```python
from build123d import *

# Parameters (mm, degrees)
SKETCH1_R          = 22
SKETCH1_R_2        = 19
OUTER_RING_DEPTH   = 8
SKETCH2_R          = 15
SKETCH2_R_2        = 9.25
HUB_DEPTH          = 8
SKETCH3_W          = 6
SKETCH3_H          = 5
SPOKES_DEPTH       = 8
SKETCH4_R          = 11
BEARING_SEAT_DEPTH = 7
SCREW_GROOVE_DEPTH = 2


with BuildPart() as part:
    # Sketch1 → Outer_ring (new body)
    with BuildSketch(Plane.XY):
        Circle(SKETCH1_R)
        Circle(SKETCH1_R_2, mode=Mode.SUBTRACT)
    extrude(amount=OUTER_RING_DEPTH)



with BuildPart() as body_2:
    # Sketch2 → Hub (new body)
    with BuildSketch(Plane.XY):
        Circle(SKETCH2_R)
        Circle(SKETCH2_R_2, mode=Mode.SUBTRACT)
    extrude(amount=HUB_DEPTH)


with BuildPart() as part_1:
    add(part.part)

    add(body_2.part)  # Spokes merges body 2
    # Sketch3 → Spokes (add)
    with BuildSketch(Plane.XY):
        Polygon((9.165063509, 10.874355653), (12.165063509, 16.070508076), (7.834936491, 18.570508076), (4.834936491, 13.374355653), align=None)
        with Locations((-17, 0)):
            Rectangle(SKETCH3_W, SKETCH3_H)
        Polygon((4.834936491, -13.374355653), (7.834936491, -18.570508076), (12.165063509, -16.070508076), (9.165063509, -10.874355653), align=None)
    extrude(amount=SPOKES_DEPTH)

    # Sketch4 → Bearing_seat (cut)
    with BuildSketch(Plane.XY):
        Circle(SKETCH4_R)
    extrude(amount=BEARING_SEAT_DEPTH, mode=Mode.SUBTRACT)

    # Sketch5 → Screw_groove (cut)
    with BuildSketch(Plane.XY.offset(3)):
        Polygon((20.820342089, -2.741050037), (20.849003007, -2.513776761), (20.875183103, -2.286204372), (20.89887926, -2.058359947), (20.92008866, -1.830270598), (20.938808778, -1.601963465), (20.955037388, -1.373465714), (20.968772558, -1.144804534), (20.980012653, -0.916007135), (20.988756337, -0.687100739), (20.995002569, -0.458112586), (20.998750605, -0.229069921), (21, 0), (20.998750605, 0.229069921), (20.995002569, 0.458112586), (20.988756337, 0.687100739), (20.980012653, 0.916007135), (20.968772558, 1.144804534), (20.955037388, 1.373465714), (20.938808778, 1.601963465), (20.92008866, 1.830270598), (20.89887926, 2.058359947), (20.875183103, 2.286204372), (20.849003007, 2.513776761), (20.820342089, 2.741050037), (23.298954242, 3.067365517), (23.298954242, -3.067365517), align=None)
    extrude(amount=SCREW_GROOVE_DEPTH, mode=Mode.SUBTRACT)


solid = part_1.part
```
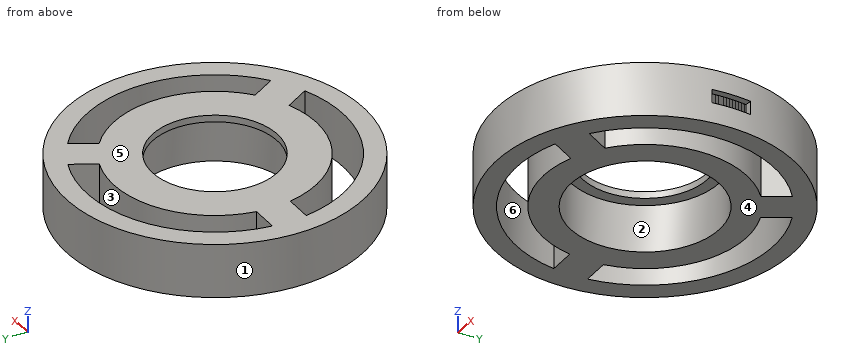
Here's how the part is built. I have some questions about the finished solid (model axes, mm). Face numbers are marked on the shaded views. A direction names the side the tool comes from. Give positions to 0.01 mm unless a question says otherwise; leave off trailing zeros. Order: outer loops, then holes, each group sorted by start corner. A loop starts at its lowest first (then second) coordinate and runs counter-clockwise, first axis right, second up. Notation, with made-up numbers: M 53.25,75 L 70.25,75 A21 ccw 70.25,112 Z; hole C 25.5,-24.75 d10. An arc over 180 degrees is marked long. Use a Markdown table: item, result. Add a question column.
1. If we mould it in two halves opening along Y, with no side actions, what happens to the marked faces 1, 2, 3 and 4? For each: +Y half, -Y half, draft (parallel to the pull), parting line (faces both ways), or undercut.
2. For pin 1 Ø2 at (x, z) = (-16.5, 2) entering from -Y; pin 2 Ø1.5 at (x, y) = (1.5, -9.5) entering from -Z; pin 3 Ø1 at (y, z) = (-15, 3) entering from +X; pin 4 Ø12 at (x, y) = (9, 2) entering from +Z, each with a flat end and sliding along its axis, tell me the tip position at first contact or that it passes through.
3. Suppose I cut it at C-C (y = -5.5). List the corners of the cut face in (x, z) for me.
4. Suppose I cut it at B-B (z = 6). List the corners of the cut face in (x, y) for me, and give its area (3 significant figures).
5. Suppose I cut it at A-A (x = 0). List the corners of the cut face in (y, z) for me.
6. On a 3-axis mill with a long thin cutter (end or side, diameter ignored), from which of +Z, -Z, +X, -X, +Y, -Y can I reach the whole of each face in a straight line? I mean the marked faces 5 and 6. Say none if no direction works.
7. I need wall thicknesses on probe 1 along Y at (x, z) = (0, 7.5); probe 2 along Y at (x, z) = (0, 3.75); probe 3 along Y at (x, z) = (-12.5, 5.75). Which ranges of each line are inside material? Lowest first, please. Write a range as from..to.
Results list:
| question | item | result |
|---|---|---|
| 1 | face 1 | parting line |
| 1 | face 2 | undercut |
| 1 | face 3 | undercut |
| 1 | face 4 | draft |
| 2 | pin 1 | stops at y = -15.61 |
| 2 | pin 2 | stops at z = 7 |
| 2 | pin 3 | stops at x = 16.55 |
| 2 | pin 4 | stops at z = 8 |
| 3 | outline | M -21.3,0 L -18.19,0 L -18.19,8 L -21.3,8 Z; M -13.96,0 L -9.53,0 L -9.53,7 L -7.44,7 L -7.44,8 L -13.96,8 Z; M 7.44,7 L 9.53,7 L 9.53,0 L 13.96,0 L 13.96,8 L 7.44,8 Z; M 18.19,0 L 21.3,0 L 21.3,8 L 18.19,8 Z |
| 4 | outline | C 0,0 d44; hole M -18.83,-2.5 A19 ccw 7.25,-17.56 L 5.23,-14.06 A15 cw -14.79,-2.5 Z; hole M -18.83,2.5 L -14.79,2.5 A15 cw 5.23,14.06 L 7.25,17.56 A19 ccw Z; hole C 0,0 d22; hole M 9.56,-11.56 L 11.58,-15.06 A19 ccw 11.58,15.06 L 9.56,11.56 A15 cw Z |
| 4 | area | 773 mm² |
| 5 | outline | M -22,0 L -19,0 L -19,8 L -22,8 Z; M -15,0 L -11,0 L -11,7 L -9.25,7 L -9.25,8 L -15,8 Z; M 9.25,7 L 11,7 L 11,0 L 15,0 L 15,8 L 9.25,8 Z; M 19,0 L 22,0 L 22,8 L 19,8 Z |
| 6 | face 5 | +Z, +X, -X, +Y, -Y |
| 6 | face 6 | +Z, -Z |
| 7 | probe 1 | y = -22..-19, -15..-9.25, 9.25..15, 19..22 |
| 7 | probe 2 | y = -22..-19, -15..-11, 11..15, 19..22 |
| 7 | probe 3 | y = -18.1..-14.31, -8.29..8.29, 14.31..18.1 |
